from build123d import *

# Parameters (mm, degrees)
SKETCH_1_R          = 4.1
EXTRUDE_1_DEPTH     = 10
FILLET_1_R          = 10
FILLET_2_R          = 14
SKETCH_5_W          = 45
SKETCH_5_H          = 8
EXTRUDE_4_DEPTH     = 42
FILLET_3_RADIUS     = 22.5
FILLET_3_LENGTH     = 8
SKETCH_6_R          = 7
SKETCH_6_R_2        = 1.6
CUT_EXTRUDE_1_DEPTH = 122.21984161
SKETCH_7_W          = 10.2
SKETCH_7_H          = 10.2
CUT_EXTRUDE_2_DEPTH = 5
SKETCH_8_R          = 1.6
CUT_EXTRUDE_3_DEPTH = 101.847657385
SKETCH_2_R          = 1.6
CUT_EXTRUDE_5_DEPTH = 101.847657385
CUT_EXTRUDE_6_REACH = 107.405
SKETCH_9_R          = 1.5
SKETCH_10_R         = 3
CUT_EXTRUDE_7_DEPTH = 2


with BuildPart() as part:
    # ｽｹｯﾁ1 → ﾎﾞｽ - 押し出し1 (new body)
    with BuildSketch(Plane(origin=(0, 0, 0), x_dir=(1, 0, 0), z_dir=(0, 1, 0))):
        Polygon((82.5, 14), (82.5, 40), (-82.5, 40), (-82.5, -40), (82.5, -40), (82.5, -14), (-7.5, -14), (-7.5, 14), align=None)
        with Locations(Location((-42.5, 0, 0), (0, 0, 270))):
            Circle(SKETCH_1_R, mode=Mode.SUBTRACT)
    extrude(amount=EXTRUDE_1_DEPTH)

    # ﾌｨﾚｯﾄ1
    fillet_1_edges = [part.edges().sort_by_distance(p)[0] for p in [
        (-82.5, 5, 40),
        (-82.5, 5, -40),
    ]]
    fillet(fillet_1_edges, radius=FILLET_1_R)

    # ﾌｨﾚｯﾄ2
    fillet_2_edges = [part.edges().sort_by_distance(p)[0] for p in [
        (-7.5, 5, -14),
        (-7.5, 5, 14),
    ]]
    fillet(fillet_2_edges, radius=FILLET_2_R - 0.0001)  # a hair under: the kernel refuses the full size

    # ｽｹｯﾁ5 → ﾎﾞｽ - 押し出し4 (add)
    with BuildSketch(Plane(origin=(0, 10, 0), x_dir=(1, 0, 0), z_dir=(0, 1, 0))):
        with Locations((25.5, 36)):
            Rectangle(SKETCH_5_W, SKETCH_5_H)
    extrude(amount=EXTRUDE_4_DEPTH)

    # ﾌｨﾚｯﾄ3: full round fillet: the end face becomes a half cylinder, R = half its width
    fillet_3_face = Plane((25.5, 52, -36), x_dir=(0, 0, -1), z_dir=(0, 1, 0))  # on the end face: x along it, z out of the body
    fillet_3_slab = fillet_3_face.offset(-FILLET_3_RADIUS / 2) * Box(FILLET_3_LENGTH, 2 * FILLET_3_RADIUS, FILLET_3_RADIUS, mode=Mode.PRIVATE)  # the body's end, R deep
    fillet_3_round = Plane((25.5, 29.5, -36), x_dir=(0, 1, 0), z_dir=(0, 0, -1)) * Cylinder(FILLET_3_RADIUS, FILLET_3_LENGTH, mode=Mode.PRIVATE)  # its axis R under the face
    add(fillet_3_slab - fillet_3_round, mode=Mode.SUBTRACT)

    # ｽｹｯﾁ6 → ｶｯﾄ - 押し出し1 (cut, through all)
    with BuildSketch(Plane.XY.offset(-32)):
        with Locations((32.5, 30)):
            Circle(SKETCH_6_R)
        with Locations((25.5, 45.5)):
            Circle(SKETCH_6_R_2)
        with Locations((38.923393759, 37.75)):
            Circle(SKETCH_6_R_2)
        with Locations((38.923393759, 22.25)):
            Circle(SKETCH_6_R_2)
        with Locations((25.5, 14.5)):
            Circle(SKETCH_6_R_2)
        with Locations((12.076606241, 22.25)):
            Circle(SKETCH_6_R_2)
        with Locations((12.076606241, 37.75)):
            Circle(SKETCH_6_R_2)
    extrude(amount=-CUT_EXTRUDE_1_DEPTH, mode=Mode.SUBTRACT)

    # ｽｹｯﾁ7 → ｶｯﾄ - 押し出し2 (cut)
    with BuildSketch(Plane(origin=(0, 10, 0), x_dir=(1, 0, 0), z_dir=(0, 1, 0))):
        with Locations((-0.5, 25)):
            Rectangle(SKETCH_7_W, SKETCH_7_H)
        with Locations((-0.5, -25)):
            Rectangle(SKETCH_7_W, SKETCH_7_H)
        with Locations((-20.5, 0)):
            Rectangle(SKETCH_7_W, SKETCH_7_H)
    extrude(amount=-CUT_EXTRUDE_2_DEPTH, mode=Mode.SUBTRACT)

    # ｽｹｯﾁ8 → ｶｯﾄ - 押し出し3 (cut, through all)
    with BuildSketch(Plane(origin=(0, 10, 0), x_dir=(1, 0, 0), z_dir=(0, 1, 0))):
        with Locations(Location((73, 27, 0), (0, 0, 270))):
            Circle(SKETCH_8_R)
        with Locations(Location((64, 27, 0), (0, 0, 270))):
            Circle(SKETCH_8_R)
        with Locations(Location((64, -27, 0), (0, 0, 270))):
            Circle(SKETCH_8_R)
        with Locations(Location((73, -27, 0), (0, 0, 270))):
            Circle(SKETCH_8_R)
    extrude(amount=-CUT_EXTRUDE_3_DEPTH, mode=Mode.SUBTRACT)

    # ｽｹｯﾁ2 → ｶｯﾄ - 押し出し5 (cut, through all)
    with BuildSketch(Plane(origin=(0, 10, 0), x_dir=(1, 0, 0), z_dir=(0, 1, 0))):
        with Locations(Location((-67.5, 25, 0), (0, 0, 270))):
            Circle(SKETCH_2_R)
        with Locations(Location((-67.5, -25, 0), (0, 0, 270))):
            Circle(SKETCH_2_R)
    extrude(amount=-CUT_EXTRUDE_5_DEPTH, mode=Mode.SUBTRACT)

    # ｽｹｯﾁ9 → ｶｯﾄ - 押し出し6 (cut, up to next)
    with BuildSketch(Plane(origin=(0, 0, 0), x_dir=(1, 0, 0), z_dir=(0, 1, 0)), mode=Mode.PRIVATE) as cut_extrude_6_sk1:
        with Locations(Location((-0.5, 25, 0), (0, 0, 270))):
            Circle(SKETCH_9_R)
    cut_extrude_6_tool1 = extrude(cut_extrude_6_sk1.sketch, amount=CUT_EXTRUDE_6_REACH, mode=Mode.PRIVATE) & part.part
    # ｽｹｯﾁ9 → ｶｯﾄ - 押し出し6 (cut, up to next)
    with BuildSketch(Plane(origin=(0, 0, 0), x_dir=(1, 0, 0), z_dir=(0, 1, 0)), mode=Mode.PRIVATE) as cut_extrude_6_sk2:
        with Locations(Location((-20.5, 0, 0), (0, 0, 90))):
            Circle(SKETCH_9_R)
    cut_extrude_6_tool2 = extrude(cut_extrude_6_sk2.sketch, amount=CUT_EXTRUDE_6_REACH, mode=Mode.PRIVATE) & part.part
    # ｽｹｯﾁ9 → ｶｯﾄ - 押し出し6 (cut, up to next)
    with BuildSketch(Plane(origin=(0, 0, 0), x_dir=(1, 0, 0), z_dir=(0, 1, 0)), mode=Mode.PRIVATE) as cut_extrude_6_sk3:
        with Locations(Location((-0.5, -25, 0), (0, 0, 270))):
            Circle(SKETCH_9_R)
    cut_extrude_6_tool3 = extrude(cut_extrude_6_sk3.sketch, amount=CUT_EXTRUDE_6_REACH, mode=Mode.PRIVATE) & part.part
    add(cut_extrude_6_tool1.solids().sort_by_distance((-0.5, 0, -25))[0], mode=Mode.SUBTRACT)
    add(cut_extrude_6_tool2.solids().sort_by_distance((-20.5, 0, 0))[0], mode=Mode.SUBTRACT)
    add(cut_extrude_6_tool3.solids().sort_by_distance((-0.5, 0, 25))[0], mode=Mode.SUBTRACT)

    # ｽｹｯﾁ10 → ｶｯﾄ - 押し出し7 (cut)
    with BuildSketch(Plane.XZ):
        with Locations(Location((-0.5, 25, 0), (0, 0, 270))):
            Circle(SKETCH_10_R)
        with Locations(Location((-20.5, 0, 0), (0, 0, 270))):
            Circle(SKETCH_10_R)
        with Locations(Location((-0.5, -25, 0), (0, 0, 270))):
            Circle(SKETCH_10_R)
        Polygon((-67.5, 28.1), (-70.184678752, 26.55), (-70.184678752, 23.45), (-67.5, 21.9), (-64.815321248, 23.45), (-64.815321248, 26.55), align=None)
        Polygon((-67.5, -21.9), (-70.184678752, -23.45), (-70.184678752, -26.55), (-67.5, -28.1), (-64.815321248, -26.55), (-64.815321248, -23.45), align=None)
    extrude(amount=-CUT_EXTRUDE_7_DEPTH, mode=Mode.SUBTRACT)


solid = part.part
The model under review builds one solid part; all positions refer to its coordinate system, in mm. A direction names the side the tool comes from. Round coordinates to 2 decimals unless told otherwise and drop trailing zeros. Write each loop counter-clockwise with the first axis right and the second up, starting at its lowest first coordinate (ties: lowest second). Pieces come first, ordered by that corner, then holes. Notation, with made-up numbers: (-35.5, -25.5) -> (-30.5, -25.5) arc R26 ccw to (-30.5, 5.5) -> close; hole circle Ø7 at (-7.75, 1). An arc over 180 degrees is marked (long way). Answer as a JSON object with one key per item and string values.
1. We need section D-D on x = 32.5. State the section outline as (y, z) points.
Results found:
{"outline": "(0, -40) -> (23, -40) -> (23, -32) -> (10, -32) -> (10, -14) -> (0, -14) -> close; (0, 14) -> (10, 14) -> (10, 40) -> (0, 40) -> close; (37, -40) -> (50.88, -40) -> (50.88, -32) -> (37, -32) -> close"}
2. We need section B-B on y = 14.5. State the section outline as (x, z) points.
Results found:
{"outline": "(3, -40) -> (23.9, -40) -> (23.9, -32) -> (3, -32) -> close; (27.1, -40) -> (48, -40) -> (48, -32) -> (27.1, -32) -> close"}
3. We need section C-C on x = -42.5. State the section outline as (y, z) points.
Results found:
{"outline": "(0, -40) -> (10, -40) -> (10, -4.1) -> (0, -4.1) -> close; (0, 4.1) -> (10, 4.1) -> (10, 40) -> (0, 40) -> close"}
4. We need section A-A on x = 73. State the section outline as (y, z) points, and give its area (3 significant figures).
Results found:
{"outline": "(0, -40) -> (10, -40) -> (10, -28.6) -> (0, -28.6) -> close; (0, -25.4) -> (10, -25.4) -> (10, -14) -> (0, -14) -> close; (0, 14) -> (10, 14) -> (10, 25.4) -> (0, 25.4) -> close; (0, 28.6) -> (10, 28.6) -> (10, 40) -> (0, 40) -> close", "area": "456 mm^2"}
5. The part is to be moulded in two halves that separate along X. For faces 6 (the face through (-5.6, 8, -25)), 7 (the face through (-82.5, 5, 0)), 8 (the face through (-19, 10, 8)), say which applies: pulls with the +X half, pulls with the -X half, needs draft (parallel to the pull), parting line crosses it, or undercut.
Results found:
{"face 6": "undercut", "face 7": "pulls with the -X half", "face 8": "needs draft"}
6. Clearance check with flat-ended pins moving along their axes: pin 1 (3.5 mm diameter, centred on x = 73, z = -27, fed in from +Y); pin 2 (4 mm diameter, centred on x = 38.92, y = 37.75, fed in from +Z); pin 3 (3 mm diameter, centred on x = -21, z = -2.5, fed in from +Y). State where each tip first meets the part, or that it passes through.
Results found:
{"pin 1": "stops at y = 10", "pin 2": "stops at z = -32", "pin 3": "stops at y = 5"}
7. To check wall thickness, follow line 1 along Z through (x, y) = (-67, 4); line 2 along X through (y, z) = (3, 0); line 3 along X through (y, z) = (6, -27). State the ranges of each line that lie inside material, in increasing order.
Results found:
{"line 1": "z = -40 to -26.52, -23.48 to 23.48, 26.52 to 40", "line 2": "x = -82.5 to -46.6, -38.4 to -22, -19 to -7.5", "line 3": "x = -82.5 to -5.6, 4.6 to 62.4, 65.6 to 71.4, 74.6 to 82.5"}
8. Machinability: for faces 1 (the face through (-0.4, 1, 28)), 2 (the face through (82.5, 5, 27)), 3 (the face through (4.6, 8, 25)), 4 (the face through (38.966, 27.319, -35.944)), 5 (the face through (-3.3, 5.1, -10)), which of the approach directions +Z, -Z, +X, -X, +Y, -Y give a long, thin tool a straight path to every point of the face, cutting with its end or side? Answer none if there is none.
Results found:
{"face 1": "-Y", "face 2": "+Z, -Z, +X, +Y, -Y", "face 3": "+Y", "face 4": "+Z, -Z", "face 5": "+X, +Y, -Y"}
